Could you check a few things on this model? Use its own coordinates, in mm. A direction names the side the tool comes from. Coordinates: 2 decimals unless noted, no trailing zeros. Loops run counter-clockwise (first coordinate to the right, second up) from the corner with the lowest first, then second, coordinate; pieces in that order, holes last. Notation, with made-up numbers: (-10.5, 34) - (3.5, 34) arc R21 cw to (3.5, 58) - close; hole circle Ø11 at (65, -14). An arc over 180 degrees is marked (long way). Use CSV: the item, a comma, the result in double quotes.
from build123d import *

# Parameters (mm, degrees)
BOSS_EXTRUDE1_DEPTH = 3
SKETCH3_W           = 3.2
SKETCH3_H           = 8.875
SKETCH3_H_2         = 8.675
SKETCH3_H_3         = 3.2
SKETCH3_W_2         = 10.2
CUT_EXTRUDE1_DEPTH  = 4
BOSS_EXTRUDE2_DEPTH = 3


with BuildPart() as part:
    # Sketch1 → Boss-Extrude1 (new body)
    with BuildSketch(Plane(origin=(0, 0, 0), x_dir=(1, 0, 0), z_dir=(0, 1, 0))):
        Polygon((15, 0), (15, 25), (95.344434203, 25), (95.344434203, 0), (110.344434203, 0), (110.344434203, 52.05), (0, 52.05), (0, 0), align=None)
    extrude(amount=-BOSS_EXTRUDE1_DEPTH)

    # Sketch3 → Cut-Extrude1 (cut, through all)
    with BuildSketch(Plane(origin=(0, 0, 0), x_dir=(1, 0, 0), z_dir=(0, 1, 0))):
        with Locations((1.5, 47.7125)):
            Rectangle(SKETCH3_W, SKETCH3_H)
        with Locations((1.5, 30.3625)):
            Rectangle(SKETCH3_W, SKETCH3_H_2)
        with Locations((1.5, 13.0125)):
            Rectangle(SKETCH3_W, SKETCH3_H_2)
        with Locations((108.844434203, 50.55)):
            Rectangle(SKETCH3_W, SKETCH3_H_3)
        with Locations((55.172217102, 50.55)):
            Rectangle(SKETCH3_W_2, SKETCH3_H_3)
        with Locations((55.172217102, 42.45)):
            Rectangle(SKETCH3_W_2, SKETCH3_H_3)
        with Locations((55.172217102, 31.5)):
            Rectangle(SKETCH3_W_2, SKETCH3_H_3)
        with Locations((35.172217102, 50.55)):
            Rectangle(SKETCH3_W_2, SKETCH3_H_3)
        with Locations((35.172217102, 42.45)):
            Rectangle(SKETCH3_W_2, SKETCH3_H_3)
        with Locations((35.172217102, 31.5)):
            Rectangle(SKETCH3_W_2, SKETCH3_H_3)
        with Locations((15.172217102, 50.55)):
            Rectangle(SKETCH3_W_2, SKETCH3_H_3)
        with Locations((15.172217102, 42.45)):
            Rectangle(SKETCH3_W_2, SKETCH3_H_3)
        with Locations((108.844434203, 13.0125)):
            Rectangle(SKETCH3_W, SKETCH3_H_2)
        with Locations((108.844434203, 30.3625)):
            Rectangle(SKETCH3_W, SKETCH3_H_2)
        with Locations((95.172217102, 50.55)):
            Rectangle(SKETCH3_W_2, SKETCH3_H_3)
        with Locations((95.172217102, 42.45)):
            Rectangle(SKETCH3_W_2, SKETCH3_H_3)
        with Locations((75.172217102, 31.5)):
            Rectangle(SKETCH3_W_2, SKETCH3_H_3)
        with Locations((75.172217102, 42.45)):
            Rectangle(SKETCH3_W_2, SKETCH3_H_3)
        with Locations((75.172217102, 50.55)):
            Rectangle(SKETCH3_W_2, SKETCH3_H_3)
    extrude(amount=-CUT_EXTRUDE1_DEPTH, mode=Mode.SUBTRACT)

    # Sketch4 → Boss-Extrude2 (add)
    with BuildSketch(Plane(origin=(0, 0, 0), x_dir=(1, 0, 0), z_dir=(0, 1, 0))):
        Polygon((95.344434203, 15), (87.344434203, 15), (87.344434203, 23), (91.344434203, 23), (91.344434203, 19), (95.344434203, 19), align=None)
    extrude(amount=-BOSS_EXTRUDE2_DEPTH)


solid = part.part
(1) Will these pins go through, and if not, where does the flat tip stop? pin 1 (0.9 mm diameter, centred on x = 109, y = -1, fed in from -Z); pin 2 (0.9 mm diameter, centred on x = 74, y = -1, fed in from +Z); pin 3 (0.9 mm diameter, centred on y = -1.5, z = -50, fed in from +X).
Computed:
pin 1,"stops at z = -48.95"
pin 2,"stops at z = -25"
pin 3,"stops at x = 107.24"
(2) Suppose I cut it at B-B (x = 76). Write out the boundary of the cut face in (y, z).
Computed:
outline,"(-3, -48.95) - (0, -48.95) - (0, -44.05) - (-3, -44.05) - close; (-3, -40.85) - (0, -40.85) - (0, -33.1) - (-3, -33.1) - close; (-3, -29.9) - (0, -29.9) - (0, -25) - (-3, -25) - close"
(3) Suppose I cut it at D-D (y = -0.85). State how many separate pieces and enclosed holes the cut face has, plus the area to 3 significant figures.
Computed:
separate pieces,"1"
enclosed holes,"8"
area,"3,220 mm²"
(4) Suppose I cut it at C-C (z = -21). Write out the boundary of the cut face in (x, y), plus the area to 3 significant figures.
Computed:
outline,"(0, -3) - (15, -3) - (15, 0) - (0, 0) - close; (87.34, -3) - (91.34, -3) - (91.34, 0) - (87.34, 0) - close; (95.34, -3) - (110.34, -3) - (110.34, 0) - (95.34, 0) - close"
area,"102 mm²"
(5) Suppose I cut it at A-A (z = -6.5). Write out the boundary of the cut face in (x, y).
Computed:
outline,"(0, -3) - (15, -3) - (15, 0) - (0, 0) - close; (95.34, -3) - (110.34, -3) - (110.34, 0) - (95.34, 0) - close"
(6) Thinking about a two-plate mould opening in X: for faces 4 (the face through (55, -1, -44.05)), 5 (the face through (65, -1, -52.05)), 6 (the face through (3.1, -1, -13)), 7 (the face through (40.272, -1, -42)), which applies, +X half, -X half, draft (parallel to the pull), parting line (faces both ways), or undercut?
Computed:
face 4,"undercut"
face 5,"draft"
face 6,"-X half"
face 7,"undercut"
(7) Please list where these lines run through material, in increasing order: line 1 (Z direction, x = 56.5, y = -2.7); line 2 (X direction, y = -0.85, z = -21.5); line 3 (Z direction, x = 92, y = -1.45).
Computed:
line 1,"z = -48.95 to -44.05, -40.85 to -33.1, -29.9 to -25"
line 2,"x = 0 to 15, 87.34 to 91.34, 95.34 to 110.34"
line 3,"z = -48.95 to -44.05, -40.85 to -25, -19 to -15"
(8) Which directions (+Z, -Z, +X, -X, +Y, -Y) give clear straight access to the entire face, cutting with the end or side of a thin tool? Please do faces 1 (the face through (109, -1, -17.35)), 2 (the face through (10.072, -1, -50)), 3 (the face through (70.072, -1, -31)).
Computed:
face 1,"+X, +Y, -Y"
face 2,"-Z, +Y, -Y"
face 3,"+Y, -Y"
